Solid Edge part; units mm, degrees
sketch "Sketch1" plane through (0, 0, 0) normal (0, 0, 1) x (1, 0, 0)
  line L0 (30, 18.5) -> (-30, 18.5)
  line L1 (-30, 18.5) -> (-30, -18.5)
  line L2 (-30, -18.5) -> (30, -18.5)
  line L3 (30, -18.5) -> (30, 18.5)
extrude "Protrusion1" add sketch "Sketch1" along normal blind 1
sketch "Sketch2" plane through (0, 0, 1) normal (0, 0, 1) x (1, 0, 0)
  circle A0 centre (-27, 16) radius 1.5
  circle A1 centre (27, 16) radius 1.5
  circle A2 centre (27, -16) radius 1.5
  circle A3 centre (-27, -16) radius 1.5
extrude "Cutout1" cut sketch "Sketch2" against normal through all
sketch "Sketch3" plane through (0, 0, 1) normal (0, 0, 1) x (1, 0, 0)
  line L0 (-23, -5) -> (-23, 5)
  line L1 (-23, 5) -> (-30, 5)
  line L2 (-30, 5) -> (-30, -5)
  line L3 (-30, -5) -> (-23, -5)
  line L4 (30, -5) -> (23, -5)
  line L5 (23, -5) -> (23, 5)
  line L6 (23, 5) -> (30, 5)
  line L7 (30, 5) -> (30, -5)
extrude "ExtrudedProtrusion_2" add sketch "Sketch3" along normal blind 10
sketch "Sketch4" plane through (0, 0, 1) normal (0, 0, 1) x (1, 0, 0)
  line L0 (9.9564, 13.8213) -> (-0.0436, 13.8213)
  line L1 (-0.0436, 13.8213) -> (-0.0436, 18.5)
  line L2 (-0.0436, 18.5) -> (9.9564, 18.5)
  line L3 (9.9564, 18.5) -> (9.9564, 13.8213)
extrude "ExtrudedProtrusion_3" add sketch "Sketch4" along normal blind 10
sketch "Sketch5" plane through (0, 0, 1) normal (0, 0, 1) x (1, 0, 0)
  circle A0 centre (18, -13.5) radius 1.5
  circle A1 centre (-18, -13.5) radius 1.5
extrude "ExtrudedProtrusion_4" add sketch "Sketch5" along normal blind 5
sketch "Sketch6" plane through (0, 0, 1) normal (0, 0, 1) x (1, 0, 0)
  line L0 (21, -16.5) -> (15, -16.5)
  line L1 (15, -16.5) -> (15, -10.5)
  line L2 (15, -10.5) -> (21, -10.5)
  line L3 (21, -10.5) -> (21, -16.5)
  line L4 (-21, -16.5) -> (-15, -16.5)
  line L5 (-15, -16.5) -> (-15, -10.5)
  line L6 (-15, -10.5) -> (-21, -10.5)
  line L7 (-21, -10.5) -> (-21, -16.5)
extrude "ExtrudedProtrusion_5" add sketch "Sketch6" along normal blind 3.5
sketch "Sketch7" plane through (0, 0, 1) normal (0, 0, 1) x (1, 0, 0)
  circle A0 centre (20, 11.5) radius 3.5
  circle A1 centre (-15.5, 11.5) radius 3.5
extrude "ExtrudedProtrusion_6" add sketch "Sketch7" along normal blind 10
sketch "Sketch8" plane through (0, 0, 1) normal (0, 0, 1) x (1, 0, 0)
  line L0 (12, -4.5) -> (-12, -4.5)
  line L1 (-12, -4.5) -> (-12, -18.5)
  line L2 (-12, -18.5) -> (12, -18.5)
  line L3 (12, -18.5) -> (12, -4.5)
extrude "ExtrudedProtrusion_7" add sketch "Sketch8" along normal blind 7
sketch "Sketch9" plane through (0, 0, 1) normal (0, 0, 1) x (1, 0, 0)
  line L0 (-2.1943, 11.4377) -> (-12, 11.4377)
  line L1 (-12, 11.4377) -> (-12, -4.5)
  line L2 (-12, -4.5) -> (-2.1943, -4.5)
  line L3 (-2.1943, -4.5) -> (-2.1943, 11.4377)
extrude "ExtrudedProtrusion_8" add sketch "Sketch9" along normal blind 10
sketch "Sketch10" plane through (0, 0, 1) normal (0, 0, 1) x (1, 0, 0)
  circle A0 centre (5, 6.5) radius 7
  circle A1 centre (5, 6.5) radius 3.9984
extrude "ExtrudedProtrusion_10" add sketch "Sketch10" along normal blind 9
sketch "Sketch11" plane through (4.9564, 16.1606, 11) normal (0, 0, 1) x (1, 0, 0)
  circle A0 centre (-3.9499, 1.4346) radius 0.7643
extrude "ExtrudedProtrusion_11" add sketch "Sketch11" along normal blind 1
chamfer "Chamfer_1" distance 2.5 angle 45 2 edges at (-23, 0, 11) (23, 0, 11)
fillet "Round_1" radius 0.5 2 edges at (16.5, 11.5, 11) (-19, 11.5, 11)
fillet "Round_2" radius 1 2 edges at (-2, 6.5, 10) (1.0016, 6.5, 10)
sketch "Sketch12" plane through (-7.0971, -4.5, 9.5) normal (0, -1, 0) x (1, 0, 0)
  line L0 (2.6971, 4.4905) -> (2.6971, -1.1067)
  arc A0 (2.6971, -1.1067) -> (3.1, -1.5095) centre (3.1, -1.1067) ccw
  line L1 (3.1, -1.5095) -> (4.0943, -1.5095)
  arc A1 (4.0943, -1.5095) -> (4.4971, -1.1067) centre (4.0943, -1.1067) ccw
  line L2 (4.4971, -1.1067) -> (4.4971, 4.4905)
  line L3 (4.4971, 4.4905) -> (2.6971, 4.4905)
  line L4 (2.0971, -1.1067) -> (2.0971, 4.4905)
  line L5 (2.0971, 4.4905) -> (0.2971, 4.4905)
  line L6 (0.2971, 4.4905) -> (0.2971, -1.1067)
  arc A2 (0.2971, -1.1067) -> (0.7, -1.5095) centre (0.7, -1.1067) ccw
  line L7 (0.7, -1.5095) -> (1.6943, -1.5095)
  arc A3 (2.0971, -1.1067) -> (1.6943, -1.5095) centre (1.6943, -1.1067) cw
  line L8 (-0.3029, -1.1067) -> (-0.3029, 4.4905)
  line L9 (-0.3029, 4.4905) -> (-2.1029, 4.4905)
  line L10 (-2.1029, 4.4905) -> (-2.1029, -1.1067)
  arc A4 (-2.1029, -1.1067) -> (-1.7, -1.5095) centre (-1.7, -1.1067) ccw
  line L11 (-1.7, -1.5095) -> (-0.7057, -1.5095)
  arc A5 (-0.7057, -1.5095) -> (-0.3029, -1.1067) centre (-0.7057, -1.1067) ccw
  line L12 (-2.7029, -1.1067) -> (-2.7029, 4.4905)
  line L13 (-2.7029, 4.4905) -> (-4.5029, 4.4905)
  line L14 (-4.5029, 4.4905) -> (-4.5029, -1.1067)
  arc A6 (-4.5029, -1.1067) -> (-4.1, -1.5095) centre (-4.1, -1.1067) ccw
  line L15 (-4.1, -1.5095) -> (-3.1057, -1.5095)
  arc A7 (-3.1057, -1.5095) -> (-2.7029, -1.1067) centre (-3.1057, -1.1067) ccw
extrude "Cutout2" cut sketch "Sketch12" against normal through all
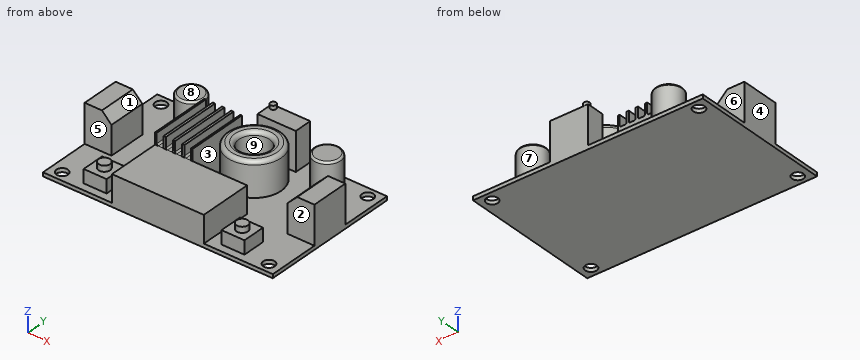
Geometry: final body of the model. Coordinates: model frame, mm. Face numbers are marked on the shaded views. A direction names the side the tool comes from. Give positions to 0.01 mm unless a question says otherwise; leave off trailing zeros. Write each loop counter-clockwise with the first axis right and the second up, starting at its lowest first coordinate (ties: lowest second). Pieces come first, ordered by that corner, then holes.
1. Line query: probe 1 along Y at (x, z) = (-27, 0.7); probe 2 along Y at (x, z) = (7.5, 4.75); probe 3 along X at (y, z) = (-14, 5.5). Output: solid intervals per line, ascending.
2. Draft query along Y for the marked faces 6, 7, 8 and 9. Return one class per face: released by +Y, released by -Y, zero draft, split by the parting line, or undercut.
3. Reachability of the marked faces 1, 2, 3, 4 and 5 from +Z, -Z, +X, -X, +Y, -Y: full face, straight path, thin tool, end or side. Return the list, or none.
4. Section query C-C, the plane y = -9.5. Return loops of the section in (x, z), then the cut area to 3 significant figures.
5. Pin query (flat end, axial travel): P1, Ø3.5, axis at x = 28, z = 4, coming from the -Y side; P2, Ø1.8, axis at y = -12, z = 2.5, coming from the +X side; P3, Ø2, axis at x = -23.5, y = 4.5, coming from the +Z side. Return the tip coordinate at first contact, or that it passes through.
6. Section query A-A, the plane y = 16. Return loops of the section in (x, z).
7. Section query B-B, the plane x = -27. Return loops of the section in (y, z).
Computed:
1. probe 1: y = -18.5 to -17.5, -14.5 to 14.5, 17.5 to 18.5
1. probe 2: y = -18.5 to -4.5, -0.04 to 3.38, 9.62 to 13.04, 13.82 to 18.5
1. probe 3: x = -19.41 to -16.59, -12 to 12, 16.59 to 19.41
2. face 6: released by +Y
2. face 7: undercut
2. face 8: zero draft
2. face 9: undercut
3. face 1: +Z, +Y, -Y
3. face 2: +Z, +X, -Y
3. face 3: +Z, +Y
3. face 4: +Z, -Z, -X, +Y, -Y
3. face 5: +Z, -X, -Y
4. outline: (-30, 0) - (30, 0) - (30, 1) - (12, 1) - (12, 8) - (-12, 8) - (-12, 1) - (-30, 1) - close
4. area: 228 mm2
5. P1: stops at y = -5
5. P2: stops at x = 21
5. P3: stops at z = 10
6. outline: (-30, 0) - (-28.5, 0) - (-28.5, 1) - (-30, 1) - close; (-25.5, 0) - (25.5, 0) - (25.5, 1) - (9.96, 1) - (9.96, 11) - (-0.04, 11) - (-0.04, 1) - (-25.5, 1) - close; (28.5, 0) - (30, 0) - (30, 1) - (28.5, 1) - close
7. outline: (-18.5, 0) - (-17.5, 0) - (-17.5, 1) - (-18.5, 1) - close; (-14.5, 0) - (14.5, 0) - (14.5, 1) - (5, 1) - (5, 11) - (-5, 11) - (-5, 1) - (-14.5, 1) - close; (17.5, 0) - (18.5, 0) - (18.5, 1) - (17.5, 1) - close
